Model file for the job. Use its own axes, mm. Face numbers are marked on the shaded views. Round coordinates to 2 decimals unless told otherwise and drop trailing zeros. Loops run counter-clockwise (first coordinate to the right, second up) from the corner with the lowest first, then second, coordinate; pieces in that order, holes last. Notation, with made-up numbers: (-28, 52) - (-14, 52) arc R23 ccw to (-14, 75) - close; hole circle Ø10 at (23.5, 41). An arc over 180 degrees is marked (long way). Answer as a JSON object with one key per item and string values.
from build123d import *

# Parameters (mm, degrees)
SKETCH1_W               = 60
SKETCH1_H               = 6.25
BOSS_EXTRUDE1_DEPTH     = 30
CUT_EXTRUDE1_DEPTH      = 68.372564891
CUT_EXTRUDE1_DEPTH_BACK = 45
CUT_EXTRUDE2_DEPTH      = 13


with BuildPart() as part:
    # Sketch1 → Boss-Extrude1 (new body)
    with BuildSketch(Plane(origin=(0, 0, 0), x_dir=(0, 0, -1), z_dir=(1, 0, 0))):
        with Locations((30, 3.125)):
            Rectangle(SKETCH1_W, SKETCH1_H)
    extrude(amount=BOSS_EXTRUDE1_DEPTH)

    # Sketch2 → Cut-Extrude1 (cut, two sides: drawn at the far end of the back side and taken through both)
    with BuildSketch(Plane.XY.offset(-CUT_EXTRUDE1_DEPTH_BACK)):
        with BuildLine():
            Line((5, 0), (25, 0))
            ThreePointArc((25, 0), (15, 4.25), (5, 0))
        make_face()
    extrude(amount=CUT_EXTRUDE1_DEPTH + CUT_EXTRUDE1_DEPTH_BACK, mode=Mode.SUBTRACT)

    # Sketch3 → Cut-Extrude2 (cut)
    with BuildSketch(Plane(origin=(0, 0, -60), x_dir=(-1, 0, 0), z_dir=(0, 0, -1))):
        Polygon((-10, 2), (-10, 5), (-20, 5), (-18.5, 3.5), (-20, 2), align=None)
    extrude(amount=-CUT_EXTRUDE2_DEPTH, mode=Mode.SUBTRACT)


solid = part.part
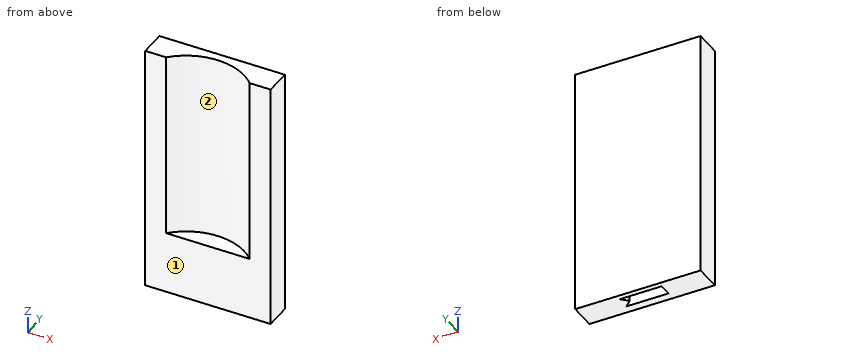
1) Slice it at A-A on z = -54. List the corners of the cut face in (x, y), then the cut area to 3 significant figures.
Values follow:
{"outline": "(0, 0) - (30, 0) - (30, 6.25) - (0, 6.25) - close; hole (10, 2) - (20, 2) - (18.5, 3.5) - (20, 5) - (10, 5) - close", "area": "160 mm²"}
2) Slice it at C-C on z = -3.5. List the corners of the cut face in (x, y), then the cut area to 3 significant figures.
Values follow:
{"outline": "(0, 0) - (5, 0) arc R13.89 cw to (25, 0) - (30, 0) - (30, 6.25) - (0, 6.25) - close", "area": "129 mm²"}
3) Slice it at D-D on x = 7. List the corners of the cut face in (y, z).
Values follow:
{"outline": "(0, -60) - (6.25, -60) - (6.25, 0) - (1.71, 0) - (1.71, -45) - (0, -45) - close"}
4) Probe probe 1 along X at (y, z) = (1.75, -20.5); probe 2 along Z at (x, y) = (10.5, 0.5); probe 3 along X at (y, z) = (2, -39.5). List the from-to ranges inside material, lowest first.
Values follow:
{"probe 1": "0 to 7.05, 22.95 to 30", "probe 2": "-60 to -45", "probe 3": "0 to 7.42, 22.58 to 30"}
5) Slice it at B-B on y = 1. List the corners of the cut face in (x, z).
Values follow:
{"outline": "(0, -60) - (30, -60) - (30, 0) - (23.93, 0) - (23.93, -45) - (6.07, -45) - (6.07, 0) - (0, 0) - close"}
6) Drop flat-ended pins along their axis: P1, Ø2, axis at x = 19.5, y = 3, coming from the +Z side; P2, Ø2, axis at x = 19, z = -21.5, coming from the -Y side; P3, Ø1.5, axis at x = 15, y = 4, coming from the -Z side. Give the stop position or say it passes through.
Values follow:
{"P1": "z = 0", "P2": "y = 3.32", "P3": "z = -47"}
7) Two-plate mould, pull along X, no slides. Class the marked faces 1 and 2: pulls with the +X half, pulls with the -X half, needs draft (parallel to the pull), parting line crosses it, or undercut.
Values follow:
{"face 1": "needs draft", "face 2": "undercut"}
